```python
from build123d import *

# Parameters (mm, degrees)
F0_W     = 30
F0_H     = 24
F1_DEPTH = 4
F2_SIZE  = 5
F3_SIZE  = 5


with BuildPart() as f1:
    # F0 (on Top) → F1 (new body)
    with BuildSketch(Plane.XY):
        Rectangle(F0_W, F0_H)
        with BuildLine():
            Line((-8.75, 1.25), (-5.25, 1.25))
            ThreePointArc((-5.25, 1.25), (-4.542893, 1.542893), (-4.25, 2.25))
            Line((-4.25, 2.25), (-4.25, 3.75))
            ThreePointArc((-4.25, 3.75), (-4.542893, 4.457107), (-5.25, 4.75))
            Line((-5.25, 4.75), (-8.75, 4.75))
            ThreePointArc((-8.75, 4.75), (-9.457107, 5.042893), (-9.75, 5.75))
            Line((-9.75, 5.75), (-9.75, 6.25))
            ThreePointArc((-9.75, 6.25), (-9.457107, 6.957107), (-8.75, 7.25))
            Line((-8.75, 7.25), (-5.25, 7.25))
            ThreePointArc((-5.25, 7.25), (-2.775126, 6.224874), (-1.75, 3.75))
            Line((-1.75, 3.75), (-1.75, -3.75))
            ThreePointArc((-1.75, -3.75), (-2.775126, -6.224874), (-5.25, -7.25))
            Line((-5.25, -7.25), (-8.75, -7.25))
            ThreePointArc((-8.75, -7.25), (-9.457107, -6.957107), (-9.75, -6.25))
            Line((-9.75, -6.25), (-9.75, -5.75))
            ThreePointArc((-9.75, -5.75), (-9.457107, -5.042893), (-8.75, -4.75))
            Line((-8.75, -4.75), (-5.25, -4.75))
            ThreePointArc((-5.25, -4.75), (-4.542893, -4.457107), (-4.25, -3.75))
            Line((-4.25, -3.75), (-4.25, -2.25))
            ThreePointArc((-4.25, -2.25), (-4.542893, -1.542893), (-5.25, -1.25))
            Line((-5.25, -1.25), (-8.75, -1.25))
            ThreePointArc((-8.75, -1.25), (-9.457107, -0.957107), (-9.75, -0.25))
            Line((-9.75, -0.25), (-9.75, 0.25))
            ThreePointArc((-9.75, 0.25), (-9.457107, 0.957107), (-8.75, 1.25))
        make_face(mode=Mode.SUBTRACT)
        with BuildLine():
            ThreePointArc((1.75, 3.75), (2.775126, 6.224874), (5.25, 7.25))
            Line((5.25, 7.25), (8.75, 7.25))
            ThreePointArc((8.75, 7.25), (9.457107, 6.957107), (9.75, 6.25))
            Line((9.75, 6.25), (9.75, 5.75))
            ThreePointArc((9.75, 5.75), (9.457107, 5.042893), (8.75, 4.75))
            Line((8.75, 4.75), (5.25, 4.75))
            ThreePointArc((5.25, 4.75), (4.542893, 4.457107), (4.25, 3.75))
            Line((4.25, 3.75), (4.25, 2.25))
            ThreePointArc((4.25, 2.25), (4.542893, 1.542893), (5.25, 1.25))
            Line((5.25, 1.25), (8.75, 1.25))
            ThreePointArc((8.75, 1.25), (9.457107, 0.957107), (9.75, 0.25))
            Line((9.75, 0.25), (9.75, -0.25))
            ThreePointArc((9.75, -0.25), (9.457107, -0.957107), (8.75, -1.25))
            Line((8.75, -1.25), (5.25, -1.25))
            ThreePointArc((5.25, -1.25), (4.542893, -1.542893), (4.25, -2.25))
            Line((4.25, -2.25), (4.25, -3.75))
            ThreePointArc((4.25, -3.75), (4.542893, -4.457107), (5.25, -4.75))
            Line((5.25, -4.75), (8.75, -4.75))
            ThreePointArc((8.75, -4.75), (9.457107, -5.042893), (9.75, -5.75))
            Line((9.75, -5.75), (9.75, -6.25))
            ThreePointArc((9.75, -6.25), (9.457107, -6.957107), (8.75, -7.25))
            Line((8.75, -7.25), (5.25, -7.25))
            ThreePointArc((5.25, -7.25), (2.775126, -6.224874), (1.75, -3.75))
            Line((1.75, -3.75), (1.75, 3.75))
        make_face(mode=Mode.SUBTRACT)
    extrude(amount=F1_DEPTH)

    # F2
    f2_edges = [f1.edges().sort_by_distance(p)[0] for p in [
        (-15, 12, 2),
    ]]
    chamfer(f2_edges, length=F2_SIZE)

    # F3
    f3_edges = [f1.edges().sort_by_distance(p)[0] for p in [
        (15, -12, 2),
    ]]
    chamfer(f3_edges, length=F3_SIZE)


solid = f1.part
```
Check sheet for the modelled part. Datum: model origin and axes. Units: mm. A direction names the side the tool comes from. Give positions to 0.01 mm unless a question says otherwise; leave off trailing zeros. Write each loop counter-clockwise with the first axis right and the second up, starting at its lowest first coordinate (ties: lowest second). Pieces come first, ordered by that corner, then holes.
Item 1: Cross-section at A-A (x = -5.75). Enter the section's corners in (y, z), and give its area (3 significant figures).
Item 2: Cross-section at C-C (y = -10.25). Enter the section's corners in (x, z), and give its area (3 significant figures).
Item 3: Draft check along Y on faces 3 (the face through (-15, -3, 2)), 4 (the face through (-7, -1.25, 2)), 5 (the face through (2.75, 6.2, 1.97)). Enter one of: released by +Y, released by -Y, zero draft, split by the parting line, or undercut.
Item 4: Cross-section at D-D (z = 3.6). Count the separate pieces of the cut face and the enclosed holes in it, and give its area (3 significant figures).
Item 5: Scan lines: L1, parallel to X at y = 3, z = 3.15; L2, parallel to X at y = 0.25, z = 0.25; L3, parallel to Y at x = 8.75, z = 3.15. Record each from-to range of solid material in increasing order.
Item 6: Cross-section at B-B (x = 3). Enter the section's corners in (y, z).
Item 7: Access from +Z, -Z, +X, -X, +Y, -Y to the whole of each face (thin tool, end or side, straight path). Record for faces 1 (the face through (9.465, 5.051, 1.972)), 2 (the face through (0, 0, 0)).
Report:
1. outline: (-12, 0) - (-7.25, 0) - (-7.25, 4) - (-12, 4) - close; (-4.75, 0) - (-1.25, 0) - (-1.25, 4) - (-4.75, 4) - close; (1.25, 0) - (4.75, 0) - (4.75, 4) - (1.25, 4) - close; (7.25, 0) - (12, 0) - (12, 4) - (7.25, 4) - close
1. area: 66.0 mm2
2. outline: (-15, 0) - (11.75, 0) - (11.75, 4) - (-15, 4) - close
2. area: 107 mm2
3. face 3: zero draft
3. face 4: undercut
3. face 5: undercut
4. separate pieces: 1
4. enclosed holes: 2
4. area: 551 mm2
5. L1: x = -15 to -4.25, -1.75 to 1.75, 4.25 to 15
5. L2: x = -15 to -9.75, -1.75 to 1.75, 9.75 to 15
5. L3: y = -12 to -7.25, -4.75 to -1.25, 1.25 to 4.75, 7.25 to 12
6. outline: (-12, 0) - (-6.43, 0) - (-6.43, 4) - (-12, 4) - close; (6.43, 0) - (12, 0) - (12, 4) - (6.43, 4) - close
7. face 1: +Z, -Z
7. face 2: -Z, +X, -X, +Y, -Y
